Input: part model. Units: mm. Frame: model coordinates. A direction names the side the tool comes from. Coordinates: 2 decimals unless noted, no trailing zeros. Order: outer loops, then holes, each group sorted by start corner. A loop starts at its lowest first (then second) coordinate and runs counter-clockwise, first axis right, second up. Notation, with made-up numbers: (87, -5.75) - (127, -5.75) arc R22 ccw to (127, 1.25) - close; hole circle Ø4 at (69, -14.5). An arc over 180 degrees is marked (long way). One line per question, with ' | ' between items. Start each with the question number.
```python
from build123d import *

# Parameters (mm, degrees)
F2_T      = -1.5
F3_R      = 80
F4_DEPTH  = 10
F5_R      = 7.5
F6_DEPTH  = 10
F7_R      = 12.5
F8_DEPTH  = 20
F10_DEPTH = 12.5
F11_R     = 7.5
F12_DEPTH = 150


with BuildPart() as f1:
    # F0 (on Front) → F1 (revolve)
    with BuildSketch(Plane.XZ):
        Polygon((10, 58.5), (0, 58.5), (0, -58.5), (47.5, -58.5), align=None)
    revolve(axis=Axis((0, 0, 0), (0, 0, 1)))

    # F2
    f2_openings = [f1.faces().sort_by_distance(p)[0] for p in [
        (0, 0, -58.5),
    ]]
    offset(amount=F2_T, openings=f2_openings)

    # F3 (on face) → F4 (join)
    with BuildSketch(Plane.XY.offset(58.5)):
        Circle(F3_R)
    extrude(amount=F4_DEPTH)

    # F5 (on face) → F6 (cut, through all)
    with BuildSketch(Plane.XY.offset(68.5)):
        with Locations((-65, 0)):
            Circle(F5_R)
        with Locations((-45.961941, -45.961941)):
            Circle(F5_R)
        with Locations((0, -65)):
            Circle(F5_R)
        with Locations((45.961941, -45.961941)):
            Circle(F5_R)
        with Locations((65, 0)):
            Circle(F5_R)
        with Locations((45.961941, 45.961941)):
            Circle(F5_R)
        with Locations((0, 65)):
            Circle(F5_R)
        with Locations((-45.961941, 45.961941)):
            Circle(F5_R)
    extrude(amount=-F6_DEPTH, mode=Mode.SUBTRACT)

    # F7 (on face) → F8 (join)
    with BuildSketch(Plane.XY.offset(68.5)):
        Circle(F7_R)
    extrude(amount=F8_DEPTH)

    # F9 (on Front) → F10 (join, symmetric)
    with BuildSketch(Plane.XZ):
        Polygon((-27.672915, 99.964498), (-18, 88.5), (18, 88.5), (18, 138.5), align=None)
    extrude(amount=F10_DEPTH, both=True)

    # F11 (on face) → F12 (join)
    with BuildSketch(Plane(origin=(0, 0, 58.5), x_dir=(1, 0, 0), z_dir=(0, 0, -1))):
        with Locations((0, -65)):
            Circle(F11_R)
        with Locations((0, 65)):
            Circle(F11_R)
    extrude(amount=-F12_DEPTH)

    # F13 (on Right) → F14 (revolve)
    with BuildSketch(Plane.YZ):
        Polygon((0, 278.771132), (-113.463566, 176.431447), (0, 176.431447), align=None)
    revolve(axis=Axis((0, 0, 227.60129), (0, 0, -1)))


solid = f1.part
```
(1) Section C-C (z = -11). Output: boundary loops of the cut face in (x, y), then the cut area to 3 significant figures.
(2) Section A-A (z = 125.5). Output: boundary loops of the cut face in (x, y), then the cut area to 3 significant figures.
(3) Reachability of faces 1 (the face through (11.923, 3.755, 78.36)), 2 (the face through (0, -12.5, 108)), 3 (the face through (-4.52, -0.18, 119.5)), 4 (the face through (-47.588, -53.284, 63.57)) from +Z, -Z, +X, -X, +Y, -Y: full face, straight path, thin tool, end or side. Return the list, or none.
(4) Section B-B (x = -65). State how many separate pieces and enclosed holes the cut face has, then the cut area to 3 significant figures.
(5) Pin query (flat end, axial travel): pin 1 (23 mm diameter, centred on x = -2, z = 105.5, fed in from -Y); pin 2 (12 mm diameter, centred on x = -89, y = 41, fed in from +Z); pin 3 (23 mm diameter, centred on x = -7, z = 114, fed in from +Y). Return the tip coordinate at first contact, or that it passes through.
(6) Material intervals for line 1 along Y through (x, z) = (-3.5, 89); line 2 along Y through (x, z) = (-65, 65); line 3 along Z through (x, y) = (12, 59.5), sorted ascending. Write a range as from..to.
(7) Draft query along Y for faces 5 (the face through (-17.34, -78.1, 63.43)), 6 (the face through (-47.59, 38.64, 63.57)), 7 (the face through (0, 12.5, 108)), 8 (the face through (18, 0, 113)). Return one class per face: +Y half, -Y half, draft (parallel to the pull), parting line (faces both ways), or undercut.
(8) Section D-D (z = 187). Output: boundary loops of the cut face in (x, y).
Worked answers:
1) outline: circle Ø64.55 at (0, 0); hole circle Ø61.4 at (0, 0) | area: 312 mm²
2) outline: circle Ø15 at (0, -65); circle Ø15 at (0, 65); (2.59, -12.5) - (18, -12.5) - (18, 12.5) - (2.59, 12.5) - close | area: 739 mm²
3) face 1: none | face 2: +X, -X | face 3: -X | face 4: -Z
4) separate pieces: 3 | enclosed holes: 0 | area: 5,900 mm²
5) pin 1: stops at y = -72.5 | pin 2: stops at z = 195.8 | pin 3: stops at y = 72.5
6) line 1: y = -71.63..-58.37, -12.5..12.5, 58.37..71.63 | line 2: y = -46.64..-7.5, 7.5..46.64 | line 3: z = 58.5..68.5, 176.43..224.02
7) face 5: parting line | face 6: undercut | face 7: undercut | face 8: draft
8) outline: circle Ø203.49 at (0, 0)
